Geometry: final body of the model. Coordinates: model frame, mm. Face numbers are marked on the shaded views. A direction names the side the tool comes from. Coordinates: 2 decimals unless noted, no trailing zeros. Order: outer loops, then holes, each group sorted by start corner. A loop starts at its lowest first (then second) coordinate and runs counter-clockwise, first axis right, second up. Notation, with made-up numbers: M 67,67.25 L 81,67.25 A12 cw 81,71.25 Z; hole C 49,63.5 d8. An arc over 180 degrees is marked long. Write item = value, one per line.
from build123d import *

# Parameters (mm, degrees)
SKETCH_1_W                       = 245
SKETCH_1_H                       = 800
SM_BASE_FLANGE_1_DEPTH           = 2
FILLET_1_R                       = 5
SKETCH_2_W                       = 1
SKETCH_2_H                       = 854.013811654
CUT_EXTRUDE_1_DEPTH              = 10
SKETCH_3_W                       = 130
SKETCH_3_H                       = 800.320249097
CUT_EXTRUDE_2_DEPTH              = 10
SM_EDGE_FLANGE_1_STRIP_W         = 9.4732
SM_EDGE_FLANGE_1_STRIP_H         = 2
SM_EDGE_FLANGE_1_STRIP_CUT_DEPTH = 800
SM_EDGE_FLANGE_1_DEPTH           = 800
FILLET_2_R                       = 5
CUT_EXTRUDE_3_DEPTH              = 10
HOLE_WIZARD_6_0_6_1_D            = 6
PATTERN_LINEAR_1_COUNT           = 6
PATTERN_LINEAR_1_PITCH           = 150


# Sheet-metal steps are written as plain solids
with BuildPart() as part:
    # Sketch 1 → 基体-法兰1 (new body)
    with BuildSketch(Plane.XY):
        Rectangle(SKETCH_1_W, SKETCH_1_H)
    extrude(amount=-SM_BASE_FLANGE_1_DEPTH)

    # 圆角1
    fillet_1_edges = [part.edges().sort_by_distance(p)[0] for p in [
        (-122.5, 400, -1),
        (122.5, 400, -1),
        (122.5, -400, -1),
        (-122.5, -400, -1),
    ]]
    fillet(fillet_1_edges, radius=FILLET_1_R)

    # Sketch 2 → 切除-拉伸1 (cut)
    with BuildSketch(Plane.XY):
        Rectangle(SKETCH_2_W, SKETCH_2_H)
    extrude(amount=-CUT_EXTRUDE_1_DEPTH, mode=Mode.SUBTRACT)


with BuildPart() as cut_extrude_1_piece_1:
    # of the separate pieces the step leaves, piece 1, a body of its own (cut_extrude_1_pieces)
    add(part.part.solids().sort_by_distance((-0.5, -400, 0))[0])

    # 边线-法兰1 strip (across the edge) → 边线-法兰1 strip cut (cut)
    with BuildSketch(Plane(origin=(-0.5, -400, 0), x_dir=(-1, 0, 0), z_dir=(0, 1, 0))):
        with Locations((-2, -1)):
            Rectangle(SM_EDGE_FLANGE_1_STRIP_W, SM_EDGE_FLANGE_1_STRIP_H)
    extrude(amount=SM_EDGE_FLANGE_1_STRIP_CUT_DEPTH, mode=Mode.SUBTRACT)

    # 边线-法兰1 section (across the edge) → 边线-法兰1 (add)
    with BuildSketch(Plane(origin=(-0.5, -400, 0), x_dir=(-1, 0, 0), z_dir=(0, 1, 0))):
        with BuildLine():
            Line((0, 0.7366), (0, 23))
            Line((0, 23), (2, 23))
            Line((2, 23), (2, 0.7366))
            ThreePointArc((2, 0.7366), (2.215745145, 0.215745145), (2.7366, 0))
            Line((2.7366, 0), (2.7366, -2))
            ThreePointArc((2.7366, -2), (0.801531583, -1.198468417), (0, 0.7366))
        make_face()
    extrude(amount=SM_EDGE_FLANGE_1_DEPTH)

    # 圆角2
    fillet_2_edges = [cut_extrude_1_piece_1.edges().sort_by_distance(p)[0] for p in [
        (-1.5, -400, 23),
        (-1.5, 400, 23),
    ]]
    fillet(fillet_2_edges, radius=FILLET_2_R)

    # 草图9 → 切除-拉伸3 (cut)
    with BuildSketch(Plane.XY):
        with BuildLine():
            Line((-99, 385), (-99, 375))
            ThreePointArc((-99, 375), (-102.5, 371.5), (-106, 375))
            Line((-106, 375), (-106, 385))
            ThreePointArc((-106, 385), (-102.5, 388.5), (-99, 385))
        make_face()
        with BuildLine():
            Line((-49, 385), (-49, 375))
            ThreePointArc((-49, 375), (-52.5, 371.5), (-56, 375))
            Line((-56, 375), (-56, 385))
            ThreePointArc((-56, 385), (-52.5, 388.5), (-49, 385))
        make_face()
        with BuildLine():
            Line((-106, -385), (-106, -375))
            ThreePointArc((-106, -375), (-102.5, -371.5), (-99, -375))
            Line((-99, -375), (-99, -385))
            ThreePointArc((-99, -385), (-102.5, -388.5), (-106, -385))
        make_face()
        with BuildLine():
            Line((-21, 375), (-21, 385))
            ThreePointArc((-21, 385), (-17.5, 388.5), (-14, 385))
            Line((-14, 385), (-14, 375))
            ThreePointArc((-14, 375), (-17.5, 371.5), (-21, 375))
        make_face()
        with BuildLine():
            Line((-14, -375), (-14, -385))
            ThreePointArc((-14, -385), (-17.5, -388.5), (-21, -385))
            Line((-21, -385), (-21, -375))
            ThreePointArc((-21, -375), (-17.5, -371.5), (-14, -375))
        make_face()
        with BuildLine():
            Line((-56, -385), (-56, -375))
            ThreePointArc((-56, -375), (-52.5, -371.5), (-49, -375))
            Line((-49, -375), (-49, -385))
            ThreePointArc((-49, -385), (-52.5, -388.5), (-56, -385))
        make_face()
    extrude(amount=-CUT_EXTRUDE_3_DEPTH, mode=Mode.SUBTRACT)

    # Ø6.0 (6) 直径孔1 (through all)
    with Locations(Plane.ZY.offset(2.5)):
        with Locations((13, 375)):
            hole_wizard_6_0_6_1 = Hole(HOLE_WIZARD_6_0_6_1_D / 2)

    # 阵列(线性)1: Ø6.0 (6) 直径孔1 ×6
    with Locations(*[(0, -i * PATTERN_LINEAR_1_PITCH, 0) for i in range(1, PATTERN_LINEAR_1_COUNT)]):
        add(hole_wizard_6_0_6_1, mode=Mode.SUBTRACT)


with BuildPart() as cut_extrude_1_piece_2:
    # of the separate pieces the step leaves, piece 2, a body of its own (cut_extrude_1_pieces)
    add(part.part.solids().sort_by_distance((117.5, -400, 0))[0])

    # Sketch 3 → 切除-拉伸2 (cut)
    with BuildSketch(Plane.XY):
        with Locations((65.5, -0.160124549)):
            Rectangle(SKETCH_3_W, SKETCH_3_H)
    extrude(amount=-CUT_EXTRUDE_2_DEPTH, mode=Mode.SUBTRACT)


solid = cut_extrude_1_piece_1.part
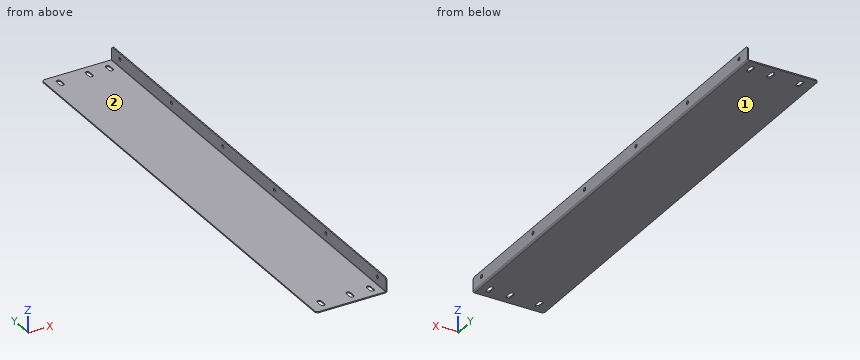
1) Line query: L1, parallel to X at y = -329.5, z = 11; L2, parallel to Z at x = -96, y = 129; L3, parallel to Z at x = -1.5, y = 225. Output: solid intervals per line, ascending.
Numbers:
L1 = -2.5 to -0.5
L2 = -2 to 0
L3 = -1.38 to 10, 16 to 23
2) Section B-B, the plane x = -79.5. Return loops of the section in (y, z).
Numbers:
outline = M -400,-2 L 400,-2 L 400,0 L -400,0 Z
3) Section A-A, the plane y = 314. Return loops of the section in (x, z).
Numbers:
outline = M -122.5,-2 L -3.24,-2 A2.74 ccw -0.5,0.74 L -0.5,23 L -2.5,23 L -2.5,0.74 A0.74 cw -3.24,0 L -122.5,0 Z
4) Set-up query: the marked faces 1 and 2. Return all of +Z, -Z, +X, -X, +Y, -Y with unobstructed straight access to the full face (end or side cutting, diameter ignored); none if empty.
Numbers:
face_1 = -Z, +X, -X, +Y, -Y
face_2 = +Z, -X, +Y, -Y
5) Pin query (flat end, axial travel): pin 1 (2 mm diameter, centred on y = -283.5, z = 18, fed in from -X); pin 2 (6 mm diameter, centred on x = -42, z = 4.5, fed in from +Y); pin 3 (8 mm diameter, centred on x = -52.5, y = -166, fed in from +Z); pin 4 (1 mm diameter, centred on y = 377.5, z = -1.5, fed in from +X). Return the tip coordinate at first contact, or that it passes through.
Numbers:
pin_1 = -2.5
pin_2 = through
pin_3 = 0
pin_4 = -1.12
